CAD build for the part. Positions are in the model's coordinates, mm. A direction names the side the tool comes from. Coordinates: 2 decimals unless noted, no trailing zeros. Order: outer loops, then holes, each group sorted by start corner. A loop starts at its lowest first (then second) coordinate and runs counter-clockwise, first axis right, second up. Notation, with made-up numbers: (56.25, -23.5) - (62.25, -23.5) arc R28 ccw to (62.25, -5.5) - close; hole circle Ø10 at (-28.5, -15). An arc over 180 degrees is marked (long way). Use one line per item in the form item = value.
```python
from build123d import *

# Parameters (mm, degrees)
SKETCH1_R           = 40
SKETCH1_R_2         = 30
BOSS_EXTRUDE1_DEPTH = 10
BOSS_EXTRUDE2_START = -1
SKETCH2_R           = 30
SKETCH2_R_2         = 27
BOSS_EXTRUDE2_DEPTH = 1
LPATTERN1_COUNT     = 2
LPATTERN1_PITCH     = 9


with BuildPart() as part:
    # Sketch1 → Boss-Extrude1 (new body)
    with BuildSketch(Plane.XY):
        Circle(SKETCH1_R)
        Circle(SKETCH1_R_2, mode=Mode.SUBTRACT)
    extrude(amount=BOSS_EXTRUDE1_DEPTH)

    # Sketch2 → Boss-Extrude2 (add)
    with BuildSketch(Plane.XY.offset(10).offset(BOSS_EXTRUDE2_START)):
        Circle(SKETCH2_R)
        Circle(SKETCH2_R_2, mode=Mode.SUBTRACT)
    boss_extrude2 = extrude(amount=BOSS_EXTRUDE2_DEPTH)

    # LPattern1: Boss-Extrude2 ×2
    with Locations(*[(0, 0, -i * LPATTERN1_PITCH) for i in range(1, LPATTERN1_COUNT)]):
        add(boss_extrude2)


solid = part.part
```
Item 1: 3-axis set-ups, long thin cutter, end or side, ignore diameter. For faces 4 (the face through (-25, 11, 1)), 5 (the face through (-5.85, -26.36, 9.49)): which of +Z, -Z, +X, -X, +Y, -Y reach the whole face in a straight line?
Derived:
face_4 = none
face_5 = +Z, -Z
Item 2: Cut at A-A, the plane y = 0. Write the cut outline in (x, z), plus the area to 3 significant figures.
Derived:
outline = (-40, 0) - (-27, 0) - (-27, 1) - (-30, 1) - (-30, 9) - (-27, 9) - (-27, 10) - (-40, 10) - close; (27, 0) - (40, 0) - (40, 10) - (27, 10) - (27, 9) - (30, 9) - (30, 1) - (27, 1) - close
area = 212 mm²
Item 3: Drill centre lines: line 1 (Y direction, x = 0, z = 0.35); line 2 (Z direction, x = -1, y = -28); line 3 (Y direction, x = 0, z = 4.25). Where is each one in solid material? Low to high. Write a range as [from, to].
Derived:
line_1 = [-40, -27], [27, 40]
line_2 = [0, 1], [9, 10]
line_3 = [-40, -30], [30, 40]
Item 4: Cut at C-C, the plane z = 3.75. Write the cut outline in (x, y), plus the area to 3 significant figures.
Derived:
outline = circle Ø80 at (0, 0); hole circle Ø60 at (0, 0)
area = 2,200 mm²
Item 5: Drop flat-ended pins along their axis: pin 1 (3 mm diameter, centred on y = -7, z = 8, fed in from -X); pin 2 (2 mm diameter, centred on x = -14, z = 4.5, fed in from -Y); pin 3 (2 mm diameter, centred on x = -25, z = 8.5, fed in from -Y). Give the stop position or say it passes through.
Derived:
pin_1 = -39.62
pin_2 = -37.83
pin_3 = -32
Item 6: Two-plate mould, pull along Z, no slides. Class faces 1 (the face through (-8.67, -39.05, 4.93)), 2 (the face through (8, -26, 0)), 3 (the face through (-25, 11, 9)): +Z half, -Z half, draft (parallel to the pull), parting line (faces both ways), or undercut.
Derived:
face_1 = draft
face_2 = -Z half
face_3 = undercut
Item 7: Cut at D-D, the plane y = -34.5. Write the cut outline in (x, z).
Derived:
outline = (-20.24, 0) - (20.24, 0) - (20.24, 10) - (-20.24, 10) - close
